For this review, take the finished solid that the model builds, in its own axes (mm). Face numbers are marked on the shaded views. A direction names the side the tool comes from. Coordinates: 2 decimals unless noted, no trailing zeros. Order: outer loops, then holes, each group sorted by start corner. A loop starts at its lowest first (then second) coordinate and runs counter-clockwise, first axis right, second up. Notation, with made-up numbers: (-4, 71.25) -> (6, 71.25) arc R26 ccw to (6, 106.25) -> close; hole circle Ø3 at (-7.5, -18). An arc over 180 degrees is marked (long way). Write item = value, one per line. Start each with the question number.
1) Consider section B-B on z = 5.25. Give the boundary of the cut face in (x, y), and give its area (3 significant figures).
2) Consider section C-C on z = 11.5. Give the boundary of the cut face in (x, y), and give its area (3 significant figures).
3) Machinability: for the marked faces 1, 2 and 3, which of the approach directions +Z, -Z, +X, -X, +Y, -Y give a long, thin tool a straight path to every point of the face, cutting with its end or side? Answer none if there is none.
4) Wall thickness on probe 1 along Y at (x, z) = (0.25, 4.5); probe 2 along Z at (x, y) = (8.25, -2.5); probe 3 along Y at (x, z) = (1, 6.75): over which ranges is each line inside the solid? List them lowest first. Write a range as [from, to].
5) Insertion check: pin 1 Ø8 at (x, y) = (0, 0) entering from +Z; pin 2 Ø8 at (y, z) = (1.5, 11.5) entering from +X; pin 3 Ø1.5 at (y, z) = (-4.5, 6.5) entering from +X; pin 4 Ø3 at (y, z) = (-2.5, 12.5) entering from -X. Each pin has a flat end and moves straight along its axis. Give the tip position at first contact, or say it passes through.
6) Consider section A-A on x = 0. Give the boundary of the cut face in (y, z), and give its area (3 significant figures).
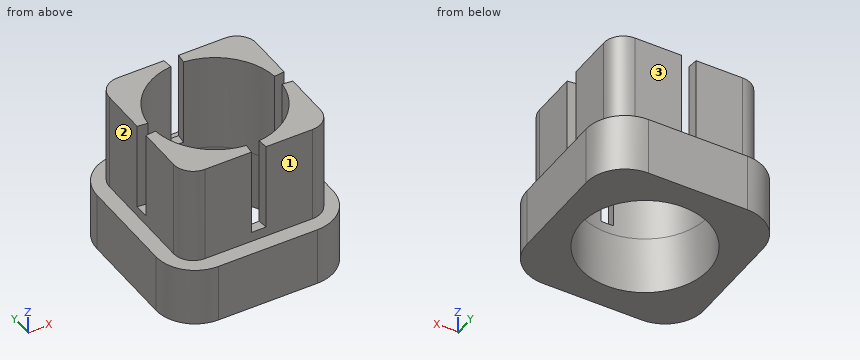
from build123d import *

# Parameters (mm, degrees)
BOSS_EXTRUDE1_DEPTH = 6
SKETCH3_R           = 6.5
BOSS_EXTRUDE2_DEPTH = 10
CUT_EXTRUDE1_DEPTH  = 9
CIRPATTERN1_COUNT   = 4
SKETCH5_R           = 6.5
CUT_EXTRUDE2_DEPTH  = 30


with BuildPart() as part:
    # Sketch1 → Boss-Extrude1 (new body)
    with BuildSketch(Plane.XY):
        with BuildLine():
            Line((-5.05, 9.05), (5.05, 9.05))
            ThreePointArc((5.05, 9.05), (7.878427125, 7.878427125), (9.05, 5.05))
            Line((9.05, 5.05), (9.05, -5.05))
            ThreePointArc((9.05, -5.05), (7.878427125, -7.878427125), (5.05, -9.05))
            Line((5.05, -9.05), (-5.05, -9.05))
            ThreePointArc((-5.05, -9.05), (-7.878427125, -7.878427125), (-9.05, -5.05))
            Line((-9.05, -5.05), (-9.05, 5.05))
            ThreePointArc((-9.05, 5.05), (-7.878427125, 7.878427125), (-5.05, 9.05))
        make_face()
    extrude(amount=BOSS_EXTRUDE1_DEPTH)

    # Sketch3 → Boss-Extrude2 (add)
    with BuildSketch(Plane.XY.offset(6)):
        with BuildLine():
            Line((-5.5, -7.5), (5.5, -7.5))
            ThreePointArc((5.5, -7.5), (6.914213562, -6.914213562), (7.5, -5.5))
            Line((7.5, -5.5), (7.5, 5.5))
            ThreePointArc((7.5, 5.5), (6.914213562, 6.914213562), (5.5, 7.5))
            Line((5.5, 7.5), (-5.5, 7.5))
            ThreePointArc((-5.5, 7.5), (-6.914213562, 6.914213562), (-7.5, 5.5))
            Line((-7.5, 5.5), (-7.5, -5.5))
            ThreePointArc((-7.5, -5.5), (-6.914213562, -6.914213562), (-5.5, -7.5))
        make_face()
        Circle(SKETCH3_R, mode=Mode.SUBTRACT)
    extrude(amount=BOSS_EXTRUDE2_DEPTH)

    # Sketch4 → Cut-Extrude1 (cut)
    with BuildSketch(Plane.XY.offset(16)):
        Polygon((0, 0), (7.5, 0.75), (7.5, -0.75), align=None)
    cut_extrude1 = extrude(amount=-CUT_EXTRUDE1_DEPTH, mode=Mode.SUBTRACT)

    # CirPattern1: Cut-Extrude1 ×4 about axis
    cirpattern1_axis = Axis((0, 0, 16), (0, 0, -1))
    for i in range(1, CIRPATTERN1_COUNT):
        add(cut_extrude1.rotate(cirpattern1_axis, i * 360 / CIRPATTERN1_COUNT), mode=Mode.SUBTRACT)

    # Sketch5 → Cut-Extrude2 (cut, symmetric)
    with BuildSketch(Plane.XY):
        with Locations(Location((0, 0, 0), (0, 0, 180))):
            Circle(SKETCH5_R)
    extrude(amount=CUT_EXTRUDE2_DEPTH, both=True, mode=Mode.SUBTRACT)


solid = part.part
Answer sheet:
q1.outline = (-9.05, -5.05) arc R4 ccw to (-5.05, -9.05) -> (5.05, -9.05) arc R4 ccw to (9.05, -5.05) -> (9.05, 5.05) arc R4 ccw to (5.05, 9.05) -> (-5.05, 9.05) arc R4 ccw to (-9.05, 5.05) -> close; hole circle Ø13 at (0, 0)
q1.area = 181 mm2
q2.outline = (-7.5, -5.5) arc R2 ccw to (-5.5, -7.5) -> (-0.75, -7.5) -> (-0.65, -6.47) arc R6.5 cw to (-6.47, -0.65) -> (-7.5, -0.75) -> close; (-7.5, 0.75) -> (-6.47, 0.65) arc R6.5 cw to (-0.65, 6.47) -> (-0.75, 7.5) -> (-5.5, 7.5) arc R2 ccw to (-7.5, 5.5) -> close; (0.65, -6.47) -> (0.75, -7.5) -> (5.5, -7.5) arc R2 ccw to (7.5, -5.5) -> (7.5, -0.75) -> (6.47, -0.65) arc R6.5 cw to start; (0.65, 6.47) arc R6.5 cw to (6.47, 0.65) -> (7.5, 0.75) -> (7.5, 5.5) arc R2 ccw to (5.5, 7.5) -> (0.75, 7.5) -> close
q2.area = 83.2 mm2
q3.face_1 = +Z, +X, -X, -Y
q3.face_2 = +Z, -X, +Y, -Y
q3.face_3 = +Z, +X, -X, +Y
q4.probe_1 = [-9.05, -6.5], [6.5, 9.05]
q4.probe_2 = [0, 6]
q4.probe_3 = [-7.5, -6.42], [6.42, 7.5]
q5.pin_1 = through
q5.pin_2 = 7.5
q5.pin_3 = 9.05
q5.pin_4 = -7.5
q6.outline = (-9.05, 0) -> (-6.5, 0) -> (-6.5, 7) -> (-7.5, 7) -> (-7.5, 6) -> (-9.05, 6) -> close; (6.5, 0) -> (9.05, 0) -> (9.05, 6) -> (7.5, 6) -> (7.5, 7) -> (6.5, 7) -> close
q6.area = 32.6 mm2
